from build123d import *


with BuildPart() as part:
    # Sketch1 → Revolve1 (revolve)
    with BuildSketch(Plane(origin=(0, 0, 0), x_dir=(1, 0, 0), z_dir=(0, 1, 0)), mode=Mode.PRIVATE) as revolve1_sk:
        with BuildLine():
            Line((0, 0), (8.255, 0))
            Line((8.255, 0), (8.255, 1.27))
            Line((8.255, 1.27), (4.826, 1.27))
            Line((4.826, 1.27), (4.826, 2.286))
            ThreePointArc((4.826, 2.286), (2.456346308, 1.606191469), (0, 1.397))
            Line((0, 1.397), (0, 0))
        make_face()
    revolve1 = revolve(revolve1_sk.sketch.rotate(Axis((0, 0, 0), (1, 0, 0)), 180), axis=Axis((0, 0, 0), (1, 0, 0)))

    # Mirror1: Revolve1 across plane
    add(revolve1.mirror(Plane(origin=(0, 0, 0), x_dir=(0, 0, 1), z_dir=(1, 0, 0))))


solid = part.part
Could you check a few things on this model? Use its own coordinates, in mm. A direction names the side the tool comes from. Give positions to 0.01 mm unless a question says otherwise; leave off trailing zeros. Write each loop counter-clockwise with the first axis right and the second up, starting at its lowest first coordinate (ties: lowest second). Pieces come first, ordered by that corner, then holes. Notation, with made-up numbers: (58.5, 47) -> (102.5, 47) arc R16 ccw to (102.5, 75) -> close; hole circle Ø4 at (22.25, -9). An arc over 180 degrees is marked (long way). Answer as CSV lines item,"result". Start each with the question number.
(1) I'm going to push flat-ended pins straight in: pin 1 Ø2 at (x, z) = (4.5, 0) entering from +Y; pin 2 Ø1 at (x, y) = (-1.5, 1) entering from +Z; pin 3 Ø1 at (y, z) = (1, 1.5) entering from +X; pin 4 Ø1.5 at (x, z) = (6.5, 0.5) entering from +Y. Where does each tip first touch, or does it pass through?
(2) Please list where these lines run through material, in increasing order: line 1 (Z direction, x = -6.75, y = 1); line 2 (Z direction, x = 0.25, y = -0.1); line 3 (Y direction, x = 4.75, z = -0.85).
(3) If we section it at B-B, the plane x = 6.25: Write out the boundary of the cut face in (y, z), and give its area (3 significant figures).
(4) If we section it at A-A, the plane y = 0: Write out the boundary of the cut face in (x, z) (3 decimals), and give its area (3 significant figures).
(5) If we section it at D-D, the plane x = -3.75: Write out the boundary of the cut face in (y, z), and give its area (3 significant figures).
(6) Which directions (+Z, -Z, +X, -X, +Y, -Y) give clear straight access to the entire face, cutting with the end or side of a thin tool? Please do faces 1 (the face through (-4.826, 0, -1.5)), 2 (the face through (4.826, 0, -1.5)), 3 (the face through (8.255, 0, 0)).
Answer list:
1,pin 1,"y = 2.29"
1,pin 2,"z = 1.39"
1,pin 3,"x = 4.83"
1,pin 4,"y = 1.27"
2,line 1,"-0.78 to 0.78"
2,line 2,"-1.39 to 1.39"
2,line 3,"-2.09 to 2.09"
3,outline,"circle Ø2.54 at (0, 0)"
3,area,"5.07 mm^2"
4,outline,"(-8.255, -1.27) -> (-4.826, -1.27) -> (-4.826, -2.286) arc R12.7 cw to (0, -1.397) arc R12.7 cw to (4.826, -2.286) -> (4.826, -1.27) -> (8.255, -1.27) -> (8.255, 1.27) -> (4.826, 1.27) -> (4.826, 2.286) arc R12.7 cw to (0, 1.397) arc R12.7 cw to (-4.826, 2.286) -> (-4.826, 1.27) -> (-8.255, 1.27) -> close"
4,area,"49.8 mm^2"
5,outline,"circle Ø3.83 at (0, 0)"
5,area,"11.5 mm^2"
6,face 1,"-X"
6,face 2,"+X"
6,face 3,"+Z, -Z, +X, +Y, -Y"
